from build123d import *

# Parameters (mm, degrees)
SKETCH1_W                  = 127.078191072
SKETCH1_H                  = 113.282646321
BOSS_EXTRUDE1_DEPTH        = 39.624
SHELL_1_T                  = -2.54
OFFICIAL_RIB_BLOCK20_REACH = 100.208


with BuildPart() as part:
    # Sketch1 → Boss-Extrude1 (new body)
    with BuildSketch(Plane(origin=(0, 0, 0), x_dir=(1, 0, 0), z_dir=(0, 1, 0))):
        with Locations((1.06119575, 7.295720781)):
            Rectangle(SKETCH1_W, SKETCH1_H)
    extrude(amount=BOSS_EXTRUDE1_DEPTH)

    # 抽壳1
    shell_1_openings = [part.faces().sort_by_distance(p)[0] for p in [
        (1.06119575, 39.624, -7.295720782),
    ]]
    offset(amount=SHELL_1_T, openings=shell_1_openings, kind=Kind.INTERSECTION)

    # 草图1 walls → official_rib_block20 (add, up to next)
    with BuildSketch(Plane(origin=(0.729572078, 0, -0.729572078), x_dir=(0.7071067811865477, 0, 0.7071067811865475), z_dir=(-0.7071067811865475, 0, 0.7071067811865477)), mode=Mode.PRIVATE) as official_rib_block20_sk1:
        Polygon((-180.846538696, -7.451602251), (-34.181409887, 32.514624019), (7.60678752, 22.77672703), (210.143173935, 50.617967106), (209.797270961, 53.134303954), (7.726, 25.357), (-34.23, 35.134), (-181.514338156, -5.000960726), align=None)
    official_rib_block20_tool1 = extrude(official_rib_block20_sk1.sketch, amount=OFFICIAL_RIB_BLOCK20_REACH, mode=Mode.PRIVATE) - part.part
    add(official_rib_block20_tool1.solids().sort_by_distance((-8.641006986, 30.2455, -10.100151142))[0])


solid = part.part
Can you work these out from the model? Positions are in its coordinate system, mm. A direction names the side the tool comes from. Coordinates: 2 decimals unless noted, no trailing zeros. Write each loop counter-clockwise with the first axis right and the second up, starting at its lowest first coordinate (ties: lowest second). Pieces come first, ordered by that corner, then holes.
Q1. Imagine slicing it at C-C, the plane z = -10. List the corners of the cut face in (x, y) for me.
Results found:
outline: (-62.48, 0) - (64.6, 0) - (64.6, 39.62) - (62.06, 39.62) - (62.06, 2.54) - (-59.94, 2.54) - (-59.94, 28.35) - (-38.34, 32.51) - (-8.54, 27.6) - (-8.54, 30.21) - (-38.41, 35.13) - (-59.94, 30.99) - (-59.94, 39.62) - (-62.48, 39.62) - close
Q2. For P1, Ø1.5, axis at x = 11, z = -39, coming from the +Y side, with a flat end and sliding along its axis, tell me the tip position at first contact or that it passes through.
Results found:
P1: stops at y = 2.54
Q3. Which directions (+Z, -Z, +X, -X, +Y, -Y) give clear straight access to the entire face, cutting with the end or side of a thin tool? Please do faces 1 (the face through (6.1, 25.9, 36.8)), 2 (the face through (-29.094, 30.177, 10.768)), 3 (the face through (-60.4, 39.624, -7.6)).
Results found:
face 1: none
face 2: +Y
face 3: +Z, -Z, +X, -X, +Y
Q4. Imagine slicing it at A-A, the plane y = 14. List the corners of the cut face in (x, z) for me, plus the area to 3 significant figures.
Results found:
outline: (-62.48, -63.94) - (64.6, -63.94) - (64.6, 49.35) - (-62.48, 49.35) - close; hole (-59.94, -61.4) - (62.06, -61.4) - (62.06, 46.81) - (-59.94, 46.81) - close
area: 1,200 mm2
Q5. Imagine slicing it at B-B, the plane x = -21.5. List the corners of the cut face in (y, z) for me.
Results found:
outline: (0, -63.94) - (39.62, -63.94) - (39.62, -61.4) - (2.54, -61.4) - (2.54, 46.81) - (24.19, 46.81) - (22.78, 32.26) - (31.88, -22.96) - (34.48, -22.96) - (25.36, 32.43) - (26.75, 46.81) - (39.62, 46.81) - (39.62, 49.35) - (0, 49.35) - close
Q6. If we mould it in two halves opening along Z, with no side actions, what happens to faces 4 (the face through (-62.478, 20, -7)), 5 (the face through (0, 20, -63.937)), 6 (the face through (-51.32, 29.77, -24.93))? For each: +Z half, -Z half, draft (parallel to the pull), parting line (faces both ways), or undercut.
Results found:
face 4: draft
face 5: -Z half
face 6: undercut
Q7. Imagine slicing it at D-D, the plane z = -53.5. List the corners of the cut face in (x, y) for me.
Results found:
outline: (-62.48, 0) - (64.6, 0) - (64.6, 39.62) - (62.06, 39.62) - (62.06, 2.54) - (-59.94, 2.54) - (-59.94, 19.97) - (-52.04, 21.49) - (-52.04, 24.13) - (-59.94, 22.6) - (-59.94, 39.62) - (-62.48, 39.62) - close
Q8. Please list where these lines run through material, in increasing order: L1, parallel to Z at x = 38.5, y = 23; L2, parallel to X at y = 11, z = -39; L3, parallel to Y at x = 26, z = 19.5.
Results found:
L1: z = -63.94 to -61.4, 46.81 to 49.35
L2: x = -62.48 to -59.94, 62.06 to 64.6
L3: y = 0 to 2.54
